```python
from build123d import *

# Parameters (mm, degrees)
BOX001027045134_W         = 10
BOX001027045134_H         = 10
BOX001027045134_DEPTH     = 32
CYLINDER192_R             = 2.2
CYLINDER192_DEPTH         = 17
CUT158_PLACEMENT_ANGLE    = 180
BOX001027045133_W         = 10
BOX001027045133_H         = 10
BOX001027045133_DEPTH     = 32
BOX001027045132_W         = 15
BOX001027045132_H         = 10
BOX001027045132_DEPTH     = 18
BOX001027045135_W         = 25
BOX001027045135_H         = 10
BOX001027045135_DEPTH     = 25
TORUS013_R                = 2.2
TORUS013_ROLL_ANGLE       = 90
COMMON091_PITCH_ANGLE     = -45
COMMON090_PLACEMENT_ANGLE = 180
CYLINDER191_R             = 2.2
CYLINDER191_DEPTH         = 9
CYLINDER193_R             = 2.2
CYLINDER193_DEPTH         = 9
CYLINDER190_R             = 1.15
CYLINDER190_DEPTH         = 32


with BuildPart() as cube187:
    # Box001027045134 → Box001027045134 (new body)
    with BuildSketch(Plane(origin=(0, -5, -22), x_dir=(1, 0, 0), z_dir=(0, 0, 1))):
        with Locations((5, 5)):
            Rectangle(BOX001027045134_W, BOX001027045134_H)
    extrude(amount=BOX001027045134_DEPTH)


with BuildPart() as cut158:
    # Cylinder192 → Cylinder192 (new body)
    with BuildSketch(Plane.XY.offset(-15)):
        Circle(CYLINDER192_R)
    extrude(amount=CYLINDER192_DEPTH)

    # Cut158: cut Cube187
    add(cube187.part, mode=Mode.SUBTRACT)


with BuildPart() as cut158_1:
    # Cut158 placement: moved
    add(cut158.part.moved(Location((0, 0, 6))).rotate(Axis((0, 0, 6), (1, 0, 0)), CUT158_PLACEMENT_ANGLE))


with BuildPart() as cube186:
    # Box001027045133 → Box001027045133 (new body)
    with BuildSketch(Plane(origin=(0, -5, -22), x_dir=(1, 0, 0), z_dir=(0, 0, 1))):
        with Locations((5, 5)):
            Rectangle(BOX001027045133_W, BOX001027045133_H)
    extrude(amount=BOX001027045133_DEPTH)


with BuildPart() as cube185:
    # Box001027045132 → Box001027045132 (new body)
    with BuildSketch(Plane(origin=(-5, -5, -18), x_dir=(1, 0, 0), z_dir=(0, 0, 1))):
        with Locations((7.5, 5)):
            Rectangle(BOX001027045132_W, BOX001027045132_H)
    extrude(amount=BOX001027045132_DEPTH)


with BuildPart() as cube188:
    # Box001027045135 → Box001027045135 (new body)
    with BuildSketch(Plane(origin=(-3, -5, -1), x_dir=(1, 0, 0), z_dir=(0, 0, 1))):
        with Locations((12.5, 5)):
            Rectangle(BOX001027045135_W, BOX001027045135_H)
    extrude(amount=BOX001027045135_DEPTH)


with BuildPart() as common090:
    # Torus013 → Torus013 (revolve)
    with BuildSketch(Plane.XZ):
        with Locations((20, 0)):
            Circle(TORUS013_R)
    revolve(axis=Axis((0, 0, 0), (0, 0, 1)))


with BuildPart() as common090_1:
    # Torus013 roll: moved
    add(common090.part.rotate(Axis((0, 0, 0), (1, 0, 0)), TORUS013_ROLL_ANGLE))


with BuildPart() as common090_2:
    # Torus013 placement: moved
    add(common090_1.part.moved(Location((20, 0, 0))))

    # Common091: intersect Cube188
    add(cube188.part, mode=Mode.INTERSECT)


with BuildPart() as common090_3:
    # Common091 pitch: moved
    add(common090_2.part.rotate(Axis((0, 0, 0), (0, 1, 0)), COMMON091_PITCH_ANGLE))


with BuildPart() as common090_4:
    # Common091 placement: moved
    add(common090_3.part.moved(Location((5.857864, 0, -14.142136))))

    # Common089: intersect Cube185
    add(cube185.part, mode=Mode.INTERSECT)

    # Common090: intersect Cube186
    add(cube186.part, mode=Mode.INTERSECT)


with BuildPart() as common090_5:
    # Common090 placement: moved
    add(common090_4.part.moved(Location((0, 0, 4))).rotate(Axis((0, 0, 4), (1, 0, 0)), COMMON090_PLACEMENT_ANGLE))


with BuildPart() as cylinder238:
    # Cylinder191 → Cylinder191 (new body)
    with BuildSketch(Plane(origin=(0, 0, 4), x_dir=(1, 0, 0), z_dir=(0, 0, -1))):
        Circle(CYLINDER191_R)
    extrude(amount=CYLINDER191_DEPTH)


with BuildPart() as cylinder240:
    # Cylinder193 → Cylinder193 (new body)
    with BuildSketch(Plane(origin=(0, 0, 33), x_dir=(1, 0, 0), z_dir=(0, 0, -1))):
        Circle(CYLINDER193_R)
    extrude(amount=CYLINDER193_DEPTH)


with BuildPart() as filament_path001:
    # Cylinder190 → Cylinder190 (new body)
    with BuildSketch(Plane(origin=(0, 0, 30), x_dir=(1, 0, 0), z_dir=(0, 0, -1))):
        Circle(CYLINDER190_R)
    extrude(amount=CYLINDER190_DEPTH)

    # Fusion112082: union Cut158, Common090, Cylinder238, Cylinder240
    add(cut158_1.part)
    add(common090_5.part)
    add(cylinder238.part)
    add(cylinder240.part)


with BuildPart() as filament_path001_1:
    # Fusion112082 placement: moved
    add(filament_path001.part.moved(Location((0, 0, 5))))


solid = filament_path001_1.part
```
Model file for the job. Use its own axes, mm. A direction names the side the tool comes from. Coordinates: 2 decimals unless noted, no trailing zeros. Order: outer loops, then holes, each group sorted by start corner. A loop starts at its lowest first (then second) coordinate and runs counter-clockwise, first axis right, second up. Notation, with made-up numbers: (39.25, -34.5) - (47.25, -34.5) arc R24 cw to (47.25, -3.5) - close; hole circle Ø4 at (61.25, 40). An arc over 180 degrees is marked (long way). Return JSON: item names as keys, results as strings. Group by question number.
1) Saw through at B-B, the plane y = 0.55. Write the cut outline in (x, z).
2) Saw through at A-A, the plane y = -1.85. Write the cut outline in (x, z), plus the area to 3 significant figures.
3) Probe line 1 (Z direction, x = -1, y = -1.7); line 2 (X direction, y = -0.1, z = 31.5); line 3 (Y direction, x = -1, z = 30). List the from-to ranges inside material, lowest first. Write a range as from..to.
4) Saw through at C-C, the plane z = 30. Write the cut outline in (x, y).
5) Tool access for faces 4 (the flat face through (0, -2, 21)), 5 (the flat face through (-1.4, 0, 26)), 6 (the flat face through (1, 1, 29)): list every direction of +Z, -Z, +X, -X, +Y, -Y with a clear straight run to the whole face (end or side of a thin tool).
6) Flat gauge pin, fed straight in: P1, Ø0.8, axis at y = 1.5, z = 19, coming from the +X side. Where does the tip first touch, or does it go through?
7) Mould opens along X. For faces 1 (the cylindrical face through (1.062, 0.44, 24.747)), 2 (the flat face through (0, 0, 0)), 3 (the cylindrical face through (-2.198, -0.097, 10.293)) say: released by +X, released by -X, zero draft, split by the parting line, or undercut.
Values found:
{
 "1": {"outline": "(-2.13, 0) - (2.13, 0) - (2.13, 9) arc R17.87 cw to (8.09, 22.32) - (5.07, 25.34) arc R22.13 ccw to (1.01, 20.36) - (1.01, 29) - (2.13, 29) - (2.13, 38) - (-2.13, 38) - (-2.13, 29) - (-1.01, 29) - (-1.01, 26) - (-2.13, 26) - close"},
 "2": {"outline": "(-1.19, 0) - (1.19, 0) - (1.19, 9) arc R18.81 cw to (7.43, 22.99) - (5.74, 24.67) arc R21.19 ccw to (0, 16) - (0, 26) - (-1.19, 26) - close; (-1.19, 29) - (1.19, 29) - (1.19, 38) - (-1.19, 38) - close", "area": "97.3 mm²"},
 "3": {"line 1": "z = 0..26, 29..38", "line 2": "x = -2.2..2.2", "line 3": "y = -1.96..1.96"},
 "4": {"outline": "circle Ø4.4 at (0, 0)"},
 "5": {"face 4": "-Y", "face 5": "-X", "face 6": "none"},
 "6": {"P1": "stops at x = 5.02"},
 "7": {"face 1": "undercut", "face 2": "zero draft", "face 3": "split by the parting line"}
}
